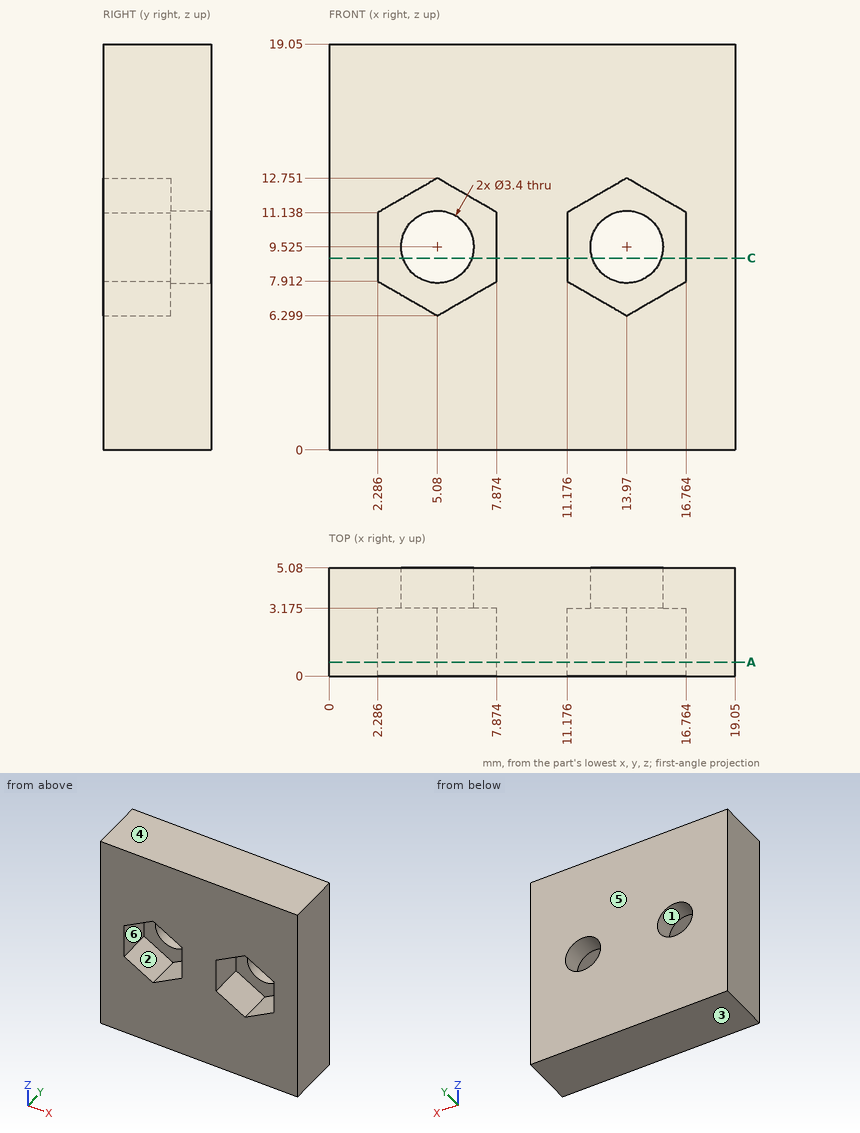
Geometry: see drawing. Coordinates: mm, zero at the bounding-box minimum. A direction names the side the tool comes from. Coordinates: 2 decimals unless noted, no trailing zeros. Loops run counter-clockwise (first coordinate to the right, second up) from the corner with the lowest first, then second, coordinate; pieces in that order, holes last. Notation, with made-up numbers: (24.5, -0.75) - (39.5, -0.75) arc R22 cw to (39.5, 35.25) - close; hole circle Ø1 at (22, 58.25). An arc over 180 degrees is marked (long way). Put each result on its own line as item: value. Start each with the question number.
Q1. Cut plane C-C, the plane z = 9. Give the number of separate pieces and of enclosed holes in the cut face.
Q2. Cut plane A-A, the plane y = 0.65. Return loops of the section in (x, z), and give its area (3 significant figures).
Q3. Pull-direction query (Z, two-part tool) for the marked faces 3, 4, 5 and 6; classes: released by +Z, released by -Z, zero draft, split by the parting line, or undercut.
Q4. Line query: line 1 (Z direction, x = 5.08, y = 3.95) (3 decimals); line 2 (X direction, y = 3.35, z = 10.5); line 3 (Y direction, x = 11.25, z = 9.5) (3 decimals). Output: solid intervals per line, ascending.
Q5. Set-up query: the marked faces 1 and 2. Return all of +Z, -Z, +X, -X, +Y, -Y with unobstructed straight access to the full face (end or side cutting, diameter ignored); none if empty.
Q6. Pin query (flat end, axial travel): pin 1 Ø4 at (x, z) = (13.97, 9.525) entering from -Y (3 decimals); pin 2 Ø3 at (y, z) = (2.5, 12.5) entering from -X; pin 3 Ø2.5 at (x, z) = (5.08, 9.525) entering from -Y. Return the tip coordinate at first contact, or that it passes through.
Filled sheet:
1. separate pieces: 3
1. enclosed holes: 0
2. outline: (0, 0) - (19.05, 0) - (19.05, 19.05) - (0, 19.05) - close; hole (2.29, 7.91) - (5.08, 6.3) - (7.87, 7.91) - (7.87, 11.14) - (5.08, 12.75) - (2.29, 11.14) - close; hole (11.18, 7.91) - (13.97, 6.3) - (16.76, 7.91) - (16.76, 11.14) - (13.97, 12.75) - (11.18, 11.14) - close
2. area: 309 mm²
3. face 3: released by -Z
3. face 4: released by +Z
3. face 5: zero draft
3. face 6: undercut
4. line 1: 0 to 7.825, 11.225 to 19.05
4. line 2: 0 to 3.69, 6.47 to 12.58, 15.36 to 19.05
4. line 3: 3.175 to 5.08
5. face 1: +Y, -Y
5. face 2: -Y
6. pin 1: y = 3.175
6. pin 2: x = 0
6. pin 3: through
